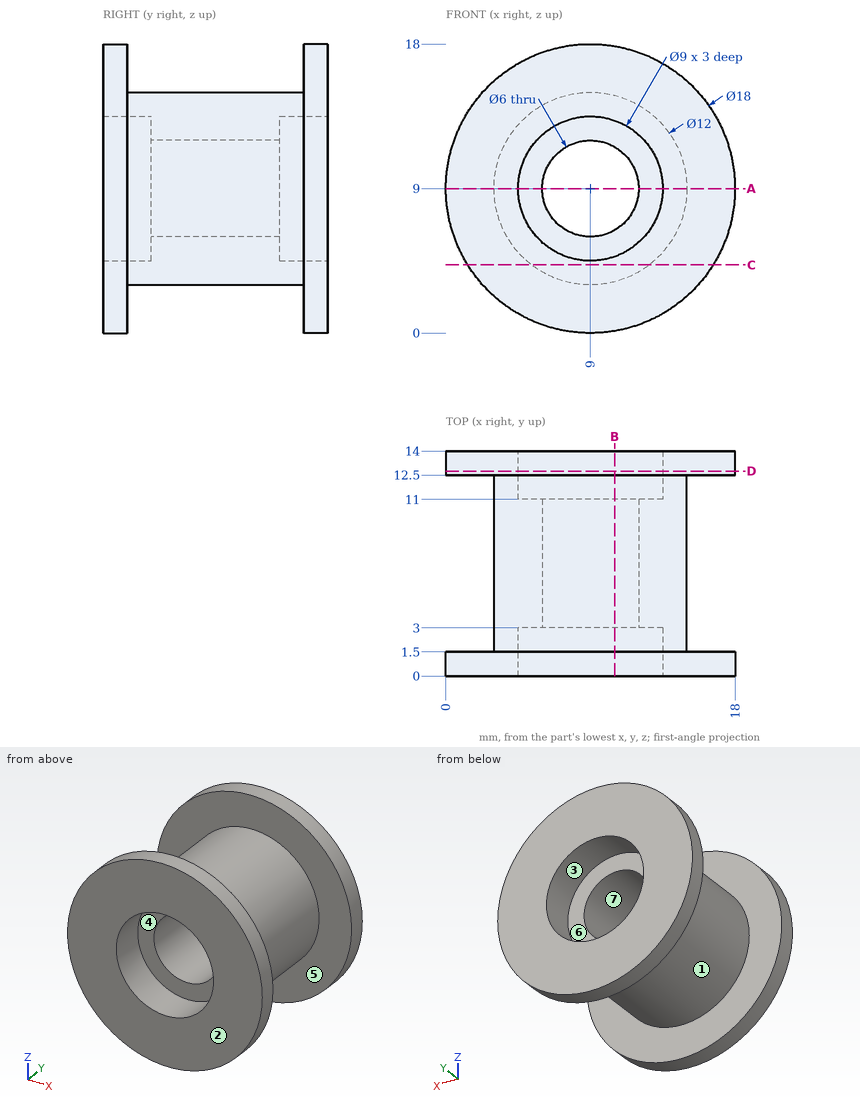
Can you work these out from the drawing? Everything is in mm from the part's minimum corner. A direction names the side the tool comes from. Round coordinates to 2 decimals unless told otherwise and drop trailing zeros. Order: outer loops, then holes, each group sorted by start corner. A loop starts at its lowest first (then second) coordinate and runs counter-clockwise, first axis right, second up. Notation, with made-up numbers: (42.25, 3.25) -> (53.25, 3.25) arc R13 cw to (53.25, 24.25) -> close; hole circle Ø11 at (59.25, 44.25). An arc over 180 degrees is marked (long way). Return JSON: item names as keys, results as strings. Group by question number.
1. If we section it at C-C, the plane z = 4.25: Write out the boundary of the cut face in (x, y), then the cut area to 3 significant figures.
2. If we section it at D-D, the plane y = 12.75: Write out the boundary of the cut face in (x, z), then the cut area to 3 significant figures.
3. Will these pins go through, and if not, where does the flat tip stop? pin 1 (7 mm diameter, centred on x = 9, z = 9, fed in from -Y); pin 2 (1.5 mm diameter, centred on y = 8.5, z = 4, fed in from +X); pin 3 (2 mm diameter, centred on y = 2, z = 14, fed in from -X); pin 4 (5.5 mm diameter, centred on x = 9, z = 5.5, fed in from -Y).
4. I need wall thicknesses on line 1 (X direction, y = 12.1, z = 9); line 2 (Y direction, x = 15.25, z = 13). Which ranges of each line are inside material? Lowest first, please. Write a range as [from, to].
5. If we section it at B-B, the plane x = 10.5: Write out the boundary of the cut face in (y, z), then the cut area to 3 significant figures.
6. We'd pull the mould along Y, two halves only. Please class the marked faces 5, 6 and 7: released by +Y, released by -Y, zero draft, split by the parting line, or undercut.
7. Which directions (+Z, -Z, +X, -X, +Y, -Y) give clear straight access to the entire face, cutting with the end or side of a thin tool? Please do the marked faces 1, 2, 3 and 4.
8. If we section it at A-A, the plane z = 9: Write out the boundary of the cut face in (x, y).
Output values:
{
 "1": {"outline": "(1.36, 0) -> (16.64, 0) -> (16.64, 1.5) -> (12.67, 1.5) -> (12.67, 12.5) -> (16.64, 12.5) -> (16.64, 14) -> (1.36, 14) -> (1.36, 12.5) -> (5.33, 12.5) -> (5.33, 1.5) -> (1.36, 1.5) -> close", "area": "127 mm²"},
 "2": {"outline": "circle Ø18 at (9, 9); hole circle Ø9 at (9, 9)", "area": "191 mm²"},
 "3": {"pin 1": "y = 3", "pin 2": "x = 13.24", "pin 3": "x = 1.01", "pin 4": "y = 0"},
 "4": {"line 1": "[3, 4.5], [13.5, 15]", "line 2": "[0, 1.5], [12.5, 14]"},
 "5": {"outline": "(0, 0.13) -> (1.5, 0.13) -> (1.5, 3.19) -> (12.5, 3.19) -> (12.5, 0.13) -> (14, 0.13) -> (14, 4.76) -> (11, 4.76) -> (11, 6.4) -> (3, 6.4) -> (3, 4.76) -> (0, 4.76) -> close; (0, 13.24) -> (3, 13.24) -> (3, 11.6) -> (11, 11.6) -> (11, 13.24) -> (14, 13.24) -> (14, 17.87) -> (12.5, 17.87) -> (12.5, 14.81) -> (1.5, 14.81) -> (1.5, 17.87) -> (0, 17.87) -> close", "area": "88.6 mm²"},
 "6": {"face 5": "undercut", "face 6": "released by +Y", "face 7": "zero draft"},
 "7": {"face 1": "none", "face 2": "+Z, -Z, +X, -X, -Y", "face 3": "+Y", "face 4": "-Y"},
 "8": {"outline": "(0, 0) -> (4.5, 0) -> (4.5, 3) -> (6, 3) -> (6, 11) -> (4.5, 11) -> (4.5, 14) -> (0, 14) -> (0, 12.5) -> (3, 12.5) -> (3, 1.5) -> (0, 1.5) -> close; (12, 3) -> (13.5, 3) -> (13.5, 0) -> (18, 0) -> (18, 1.5) -> (15, 1.5) -> (15, 12.5) -> (18, 12.5) -> (18, 14) -> (13.5, 14) -> (13.5, 11) -> (12, 11) -> close"}
}
